Can you work these out from the model? Positions are in its coordinate system, mm. A direction names the side the tool comes from. Coordinates: 2 decimals unless noted, no trailing zeros. Put each result on its own line as item: value. Start each with the question number.
from build123d import *

# Parameters (mm, degrees)
SKETCH2_R           = 6.5
BOSS_EXTRUDE1_DEPTH = 8
CUT_EXTRUDE1_DEPTH  = 13.186057607
CIRPATTERN1_COUNT   = 12


with BuildPart() as part:
    # Sketch2 → Boss-Extrude1 (new body)
    with BuildSketch(Plane.XY):
        Circle(SKETCH2_R)
        with BuildLine():
            Line((-0.9, 2.116601049), (-0.9, 1.05))
            ThreePointArc((-0.9, 1.05), (-0.943933983, 0.943933983), (-1.05, 0.9))
            Line((-1.05, 0.9), (-2.116601049, 0.9))
            ThreePointArc((-2.116601049, 0.9), (-2.3, 0), (-2.116601049, -0.9))
            Line((-2.116601049, -0.9), (-1.05, -0.9))
            ThreePointArc((-1.05, -0.9), (-0.943933983, -0.943933983), (-0.9, -1.05))
            Line((-0.9, -1.05), (-0.9, -2.116601049))
            ThreePointArc((-0.9, -2.116601049), (0, -2.3), (0.9, -2.116601049))
            Line((0.9, -2.116601049), (0.9, -1.05))
            ThreePointArc((0.9, -1.05), (0.943933983, -0.943933983), (1.05, -0.9))
            Line((1.05, -0.9), (2.116601049, -0.9))
            ThreePointArc((2.116601049, -0.9), (2.3, 0), (2.116601049, 0.9))
            Line((2.116601049, 0.9), (1.05, 0.9))
            ThreePointArc((1.05, 0.9), (0.943933983, 0.943933983), (0.9, 1.05))
            Line((0.9, 1.05), (0.9, 2.116601049))
            ThreePointArc((0.9, 2.116601049), (0, 2.3), (-0.9, 2.116601049))
        make_face(mode=Mode.SUBTRACT)
    extrude(amount=BOSS_EXTRUDE1_DEPTH)

    # Sketch3 → Cut-Extrude1 (cut, through all)
    with BuildSketch(Plane.XY.offset(8)):
        Polygon((-0.875, 6.5), (-0.5, 4.94), (0, 4.94), (0.5, 4.94), (0.875, 6.5), align=None)
    cut_extrude1 = extrude(amount=-CUT_EXTRUDE1_DEPTH, mode=Mode.SUBTRACT)

    # CirPattern1: Cut-Extrude1 ×12 about axis
    cirpattern1_axis = Axis((0, 0, 0), (0, 0, 1))
    for i in range(1, CIRPATTERN1_COUNT):
        add(cut_extrude1.rotate(cirpattern1_axis, i * 360 / CIRPATTERN1_COUNT), mode=Mode.SUBTRACT)

    # Sketch4 → Cut-Revolve1 (revolve, cut)
    with BuildSketch(Plane(origin=(0, 0, 0), x_dir=(1, 0, 0), z_dir=(0, 1, 0))):
        Polygon((-6.812692974, -8.45), (-6.812692974, -6.53), (-4.85, -8.45), align=None)
        Polygon((-4.85, 0.45), (-6.812692974, 0.45), (-6.812692974, -1.47), align=None)
    revolve(axis=Axis((0, 0, -4.663745267), (0, 0, 1)), mode=Mode.SUBTRACT)


solid = part.part
Q1. Will these pins go through, and if not, where does the flat tip stop? pin 1 (0.8 mm diameter, centred on x = 0, z = 4, fed in from -Y); pin 2 (0.9 mm diameter, centred on x = 1.5, z = 2.5, fed in from -Y); pin 3 (0.5 mm diameter, centred on x = 0, z = 5.5, fed in from +Y).
Q2. On a 3-axis mill with a long thin cutter (end or side, diameter ignored), from which of +Z, -Z, +X, -X, +Y, -Y can I reach the whole of each face in a straight line? I mean faces 1 (the cylindrical face through (0, -2.3, 3.9)), 2 (the flat face through (-0.678, -5.681, 4.056)), 3 (the conical face through (-5.69, 1.54, 0.57)), 4 (the flat face through (-4.581, 3.428, 4.056)), 5 (the conical face through (4.161, -4.178, 7.426)). Say none if no direction works.
Q3. We'd pull the mould along X, two halves only. Please class faces 6 (the conical face through (-5.69, 1.54, 7.43)), 7 (the flat face through (1.6, 0.9, 3.9)), 8 (the flat face through (-1.6, -0.9, 3.9)), 9 (the cylindrical face through (6.275, -1.694, 3.96)): released by +X, released by -X, zero draft, split by the parting line, or undercut.
Q4. Please list where these lines run through material, in increasing order: line 1 along X through (y, z) = (-5, 3.25); line 2 along Y through (x, z) = (0, 4.5); line 3 along X through (y, z) = (4.5, 1). Write a range as [from, to].
Calculated:
1. pin 1: y = -4.94
1. pin 2: y = -6.41
1. pin 3: y = 4.94
2. face 1: +Z, -Z
2. face 2: +Z, -Z, -Y
2. face 3: -Z, -X, +Y
2. face 4: +Z, -Z, -X
2. face 5: +Z, +X, -Y
3. face 6: released by -X
3. face 7: undercut
3. face 8: undercut
3. face 9: released by +X
4. line 1: [-4.15, -3.83], [-2.18, -0.51], [0.51, 2.18], [3.83, 4.15]
4. line 2: [-4.94, -2.3], [2.3, 4.94]
4. line 3: [-4.46, -3.35], [-2.09, 2.09], [3.35, 4.46]
